from build123d import *

# Parameters (mm, degrees)
SKETCH1_W                 = 60.325
SKETCH1_H                 = 12.7
BOSS_EXTRUDE1_DEPTH       = 6.35
F_4_CLEARANCE_HOLE1_D     = 3.2639
F_4_CLEARANCE_HOLE1_DEPTH = 12.7
F_4_CLEARANCE_HOLE1_TIP   = 0.980574487


with BuildPart() as part:
    # Sketch1 → Boss-Extrude1 (new body)
    with BuildSketch(Plane.XY):
        Rectangle(SKETCH1_W, SKETCH1_H)
    extrude(amount=BOSS_EXTRUDE1_DEPTH)

    # #4 Clearance Hole1
    with Locations(Plane.XY.offset(6.35)):
        with Locations((-25.4, 0), (23.8125, 0)):
            Hole(F_4_CLEARANCE_HOLE1_D / 2, depth=F_4_CLEARANCE_HOLE1_DEPTH)
            with Locations((0, 0, -(F_4_CLEARANCE_HOLE1_DEPTH + F_4_CLEARANCE_HOLE1_TIP / 2))):  # 118° drill point
                Cone(0, F_4_CLEARANCE_HOLE1_D / 2, F_4_CLEARANCE_HOLE1_TIP, mode=Mode.SUBTRACT)


solid = part.part
The listing builds one solid part. Answer for the finished solid, in the listing's coordinates (mm). Give positions to 0.01 mm unless a question says otherwise; leave off trailing zeros. Write each loop counter-clockwise with the first axis right and the second up, starting at its lowest first coordinate (ties: lowest second). Pieces come first, ordered by that corner, then holes. Notation, with made-up numbers: (-8.75, -5.75) - (19.25, -5.75) arc R17 ccw to (19.25, 0.25) - close; hole circle Ø9 at (-5.75, 29.25). An arc over 180 degrees is marked (long way). One line per question, with ' | ' between items. Start each with the question number.
1. Straight lines are drawn through the part: line 1 (X direction, y = -1.25, z = 4); line 2 (X direction, y = -1, z = 1.5); line 3 (Y direction, x = -25.4, z = 4). For each, find the intervals that lie inside material, in ascending order.
2. Determine the mould class of faces 1 (the face through (-26.957, 0.49, 3.131)), 2 (the face through (22.256, 0.49, 3.131)), 3 (the face through (0, 6.35, 3)), 4 (the face through (-30.162, 0, 3)) for opening direction X: +X half, -X half, draft (parallel to the pull), parting line (faces both ways), or undercut.
3. Section B-B, the plane x = -25.4 is taken. Determine the outline of the cut face in (y, z), then the cut area to 3 significant figures.
4. Given P1, Ø3, axis at x = 16.5, y = 3, coming from the -Z side, flat-ended and moving along its own axis, determine where the tip first touches the part or whether it passes through.
5. Section C-C, the plane z = 1.75 is taken. Determine the outline of the cut face in (x, y), then the cut area to 3 significant figures.
6. Section A-A, the plane y = 0 is taken. Determine the outline of the cut face in (x, z).
Result:
1) line 1: x = -30.16 to -26.45, -24.35 to 22.76, 24.86 to 30.16 | line 2: x = -30.16 to -26.69, -24.11 to 22.52, 25.1 to 30.16 | line 3: y = -6.35 to -1.63, 1.63 to 6.35
2) face 1: undercut | face 2: undercut | face 3: draft | face 4: -X half
3) outline: (-6.35, 0) - (-1.63, 0) - (-1.63, 6.35) - (-6.35, 6.35) - close; (1.63, 0) - (6.35, 0) - (6.35, 6.35) - (1.63, 6.35) - close | area: 59.9 mm2
4) P1: stops at z = 0
5) outline: (-30.16, -6.35) - (30.16, -6.35) - (30.16, 6.35) - (-30.16, 6.35) - close; hole circle Ø3.26 at (-25.4, 0); hole circle Ø3.26 at (23.81, 0) | area: 749 mm2
6) outline: (-30.16, 0) - (-27.03, 0) - (-27.03, 6.35) - (-30.16, 6.35) - close; (-23.77, 0) - (22.18, 0) - (22.18, 6.35) - (-23.77, 6.35) - close; (25.44, 0) - (30.16, 0) - (30.16, 6.35) - (25.44, 6.35) - close
